Work out the finished part from the listing and answer in its coordinate system (mm). Face numbers are marked on the shaded views. Coordinates: 2 decimals unless noted, no trailing zeros. Order: outer loops, then holes, each group sorted by start corner. A loop starts at its lowest first (then second) coordinate and runs counter-clockwise, first axis right, second up. Notation, with made-up numbers: M 13,-35.5 L 18,-35.5 A11 cw 18,-27.5 Z; hole C 42,80 d4. An arc over 180 degrees is marked long. Use a Markdown table: item, result.
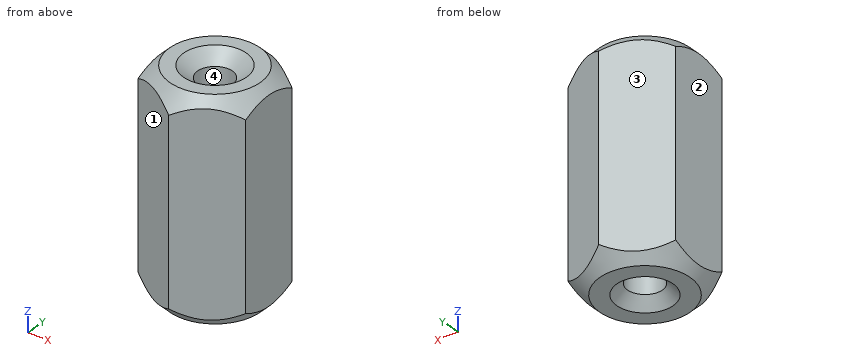
from build123d import *

# Parameters (mm, degrees)
BOSS_EXTRUDE1_DEPTH      = 6.35
BOSS_EXTRUDE1_DEPTH_BACK = 6.35


with BuildPart() as part:
    # Sketch1 → Boss-Extrude1 (new body, two sides)
    with BuildSketch(Plane.XY) as boss_extrude1_sk:
        Polygon((3.175, -1.833087105), (3.175, 1.833087105), (0, 3.666174209), (-3.175, 1.833087105), (-3.175, -1.833087105), (0, -3.666174209), align=None)
    extrude(amount=BOSS_EXTRUDE1_DEPTH)
    extrude(boss_extrude1_sk.sketch, amount=-BOSS_EXTRUDE1_DEPTH_BACK)

    # Sketch3 → Cut-Revolve2 (revolve, cut)
    with BuildSketch(Plane(origin=(0, 0, 0), x_dir=(0, 0, -1), z_dir=(1, 0, 0))):
        Polygon((-5.35, 3.666174209), (-6.35, 2.666174209), (-6.35, 3.666174209), align=None)
    cut_revolve2 = revolve(axis=Axis((0, 0, -0.635), (0, 0, 1)), mode=Mode.SUBTRACT)

    # Mirror1: Cut-Revolve2 across plane
    add(cut_revolve2.mirror(Plane.XY), mode=Mode.SUBTRACT)

    # Sketch4 → CSK for _1 Flat Head Machine Screw _100 (revolve, cut)
    with BuildSketch(Plane(origin=(0, 0, 6.35), x_dir=(0, -1, 0), z_dir=(1, 0, 0))):
        Polygon((0, 0), (0, 12.7), (1.6637, 12.7), (1.0287, 12.065), (1.0287, 0.692676746), (1.8542, 0), align=None)
    revolve(axis=Axis((0, 0, 12.7), (0, 0, -1)), mode=Mode.SUBTRACT)


solid = part.part
1. For a pull along Y with two mould halves and no side action, classify the marked faces 1, 2, 3 and 4 as +Y half, -Y half, draft (parallel to the pull), parting line (faces both ways), or undercut.
Answers below:
| item | result |
|---|---|
| face 1 | -Y half |
| face 2 | draft |
| face 3 | +Y half |
| face 4 | undercut |
2. Section B-B on y = 0 is taken. Determine the outline of the cut face in (x, z) (3 decimals).
Answers below:
| item | result |
|---|---|
| outline | M -3.175,-5.841 L -2.666,-6.35 L -1.664,-6.35 L -1.029,-5.715 L -1.029,5.657 L -1.854,6.35 L -2.666,6.35 L -3.175,5.841 Z; M 1.029,-5.715 L 1.664,-6.35 L 2.666,-6.35 L 3.175,-5.841 L 3.175,5.841 L 2.666,6.35 L 1.854,6.35 L 1.029,5.657 Z |
3. Section A-A on z = -4.25 is taken. Determine the outline of the cut face in (x, y) (3 decimals), then the cut area to 3 significant figures.
Answers below:
| item | result |
|---|---|
| outline | M -3.175,-1.833 L 0,-3.666 L 3.175,-1.833 L 3.175,1.833 L 0,3.666 L -3.175,1.833 Z; hole C 0,0 d2.057 |
| area | 31.6 mm² |
4. Find the intervals of material crossed by probe 1 along X at (y, z) = (0, -0.25) (3 decimals); probe 2 along Y at (x, z) = (-0.75, 5.25); probe 3 along Y at (x, z) = (0.5, 1.75), in increasing order.
Answers below:
| item | result |
|---|---|
| probe 1 | -3.175 to -1.029, 1.029 to 3.175 |
| probe 2 | -3.23 to -0.7, 0.7 to 3.23 |
| probe 3 | -3.38 to -0.9, 0.9 to 3.38 |
